Read the model definition and answer for the solid it produces. Units are mm, in the model's axes. Face numbers are marked on the shaded views. A direction names the side the tool comes from. Give positions to 0.01 mm unless a question says otherwise; leave off trailing zeros. Loops run counter-clockwise (first coordinate to the right, second up) from the corner with the lowest first, then second, coordinate; pieces in that order, holes last. Notation, with made-up numbers: (-23, -11.5) - (35, -11.5) arc R21 cw to (35, 12.5) - close; hole circle Ø3 at (21, 65). An arc over 180 degrees is marked (long way). Put each result on its own line as item: value. Start each with the question number.
1. Given pin 1 Ø2 at (x, y) = (166.5, -0.5) entering from -Z; pin 2 Ø2 at (y, z) = (625, 187) entering from -X; pin 3 Ø8 at (y, z) = (-83, 530) entering from +X; pin 4 Ø5 at (x, z) = (300, 183.5) entering from +Y, each flat-ended and moving along its own axis, determine where each tip first touches the part or whether it passes through.
2. A cutting plane is placed at A-A, the plane z = 88.5. Determine the outline of the cut face in (x, y), plus the area to 4 significant figures.
3. A cutting plane is placed at C-C, the plane x = -239. Determine the outline of the cut face in (y, z).
4. For the marked faces 1, 2, 3 and 4, determine the directions among +Z, -Z, +X, -X, +Y, -Y from which every point of the face is accessible in a straight line to the end or side of a thin tool.
5. A cutting plane is placed at B-B, the plane y = 500.5. Determine the outline of the cut face in (x, z).
6. Consider L1, parallel to Y at x = -165.5, z = 517; L2, parallel to X at y = 513.5, z = 349.5; L3, parallel to X at y = 179.5, z = 67. Determine where each line is inside the solid, lowest interval first. Write a range as from..to.
```python
from build123d import *

# Parameters (mm, degrees)
F2_DEPTH = 127
F4_DEPTH = 609.6


with BuildPart() as f2:
    # F1 (on Top) → F2 (new body)
    with BuildSketch(Plane.XY):
        Polygon((422.536999, 742.405157), (-466.463001, 742.405157), (-466.463001, -242.869017), (422.536999, -242.869017), (422.536999, -39.669017), (371.736999, -39.669017), (371.736999, -192.069017), (-415.663001, -192.069017), (-415.663001, 691.605157), (371.736999, 691.605157), (371.736999, 539.205157), (422.536999, 539.205157), align=None)
    extrude(amount=F2_DEPTH)

    # F3 (on face) → F4 (join)
    with BuildSketch(Plane(origin=(0, 0, 0), x_dir=(1, 0, 0), z_dir=(0, 0, -1))):
        Polygon((371.736999, 39.669017), (371.736999, 192.069017), (-415.663001, 192.069017), (-415.663001, -691.605157), (371.736999, -691.605157), (371.736999, -539.205157), align=None)
    extrude(amount=-F4_DEPTH)


solid = f2.part
```
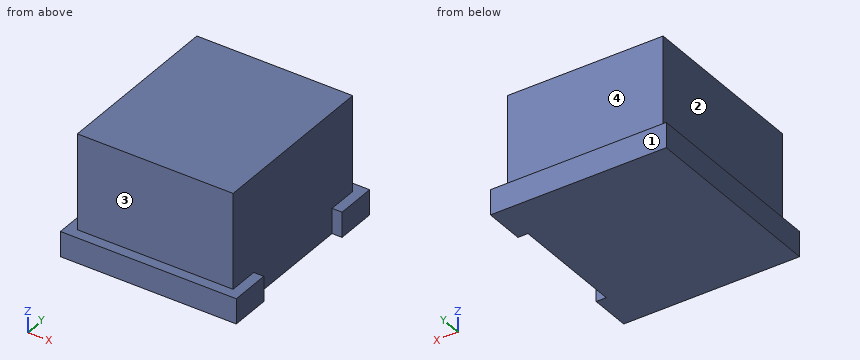
Return value:
1. pin 1: stops at z = 0
1. pin 2: stops at x = -415.66
1. pin 3: stops at x = 371.74
1. pin 4: stops at y = 691.61
2. outline: (-466.46, -242.87) - (422.54, -242.87) - (422.54, -39.67) - (371.74, -39.67) - (371.74, 539.21) - (422.54, 539.21) - (422.54, 742.41) - (-466.46, 742.41) - close
2. area: 846,500 mm2
3. outline: (-242.87, 0) - (742.41, 0) - (742.41, 127) - (691.61, 127) - (691.61, 609.6) - (-192.07, 609.6) - (-192.07, 127) - (-242.87, 127) - close
4. face 1: +Z, -Z, +X, -X, +Y
4. face 2: +Z, -X, +Y, -Y
4. face 3: +Z, +X, -X, -Y
4. face 4: +Z, +X, -X, +Y
5. outline: (-466.46, 0) - (371.74, 0) - (371.74, 609.6) - (-415.66, 609.6) - (-415.66, 127) - (-466.46, 127) - close
6. L1: y = -192.07..691.61
6. L2: x = -415.66..371.74
6. L3: x = -466.46..371.74
